Geometry: final body of the model. Coordinates: model frame, mm. A direction names the side the tool comes from. Give positions to 0.01 mm unless a question says otherwise; leave off trailing zeros. Loops run counter-clockwise (first coordinate to the right, second up) from the corner with the lowest first, then second, coordinate; pieces in that order, holes last.
Autodesk Inventor part; units mm, degrees
ref_plane "YZ Plane" through (0, 0, 0) normal (1, 0, 0) x (0, 1, 0)
ref_plane "XZ Plane" through (0, 0, 0) normal (0, 1, 0) x (-1, 0, 0)
ref_plane "XY Plane" through (0, 0, 0) normal (0, 0, 1) x (1, 0, 0)
sketch "Sketch1" plane through (0, 0, 0) normal (1, 0, 0) x (0, 1, 0)
  circle A0 centre (0, 0) radius 50.8
  circle A1 centre (0, 0) radius 3.175
  circle A2 centre (0, -31.75) radius 9.525
  line L0 (0, 0) -> (0, -74.7092) construction
  circle A3 centre (27.4963, -15.875) radius 9.525
  circle A4 centre (27.4963, 15.875) radius 9.525
  circle A5 centre (0, 31.75) radius 9.525
  circle A6 centre (-27.4963, 15.875) radius 9.525
  circle A7 centre (-27.4963, -15.875) radius 9.525
  circle A8 centre (0, -12.7) radius 3.175
  circle A9 centre (12.7, 0) radius 3.175
  circle A10 centre (0, 12.7) radius 3.175
  circle A11 centre (-12.7, 0) radius 3.175
  dimension "d0" = 101.6
  dimension "d1" = 6.35
  dimension "d2" = 19.05
  dimension "d3" = 31.75
  dimension "d6" = 360
  dimension "d16" = 6.35
  dimension "d17" = 12.7
  dimension "d24" = 360
extrude "Extrusion3" add sketch "Sketch1" along normal blind 12.7
sketch "Sketch4" plane through (0, 0, 0) normal (-1, 0, 0) x (0, 0, 1)
  circle A0 centre (0, 0) radius 6.35
  circle A1 centre (0, 0) radius 3.175
  dimension "d28" = 12.7
  dimension "d31" = 6.35
extrude "Extrusion5" add sketch "Sketch4" along normal blind 6.35
sketch "Sketch5" plane through (0, 0, 0) normal (0, 1, 0) x (-1, 0, 0)
  circle A0 centre (3.175, 0) radius 1.5875
  line L0 (0, 0) -> (21.9133, 0) construction
  line L1 (6.35, -6.35) -> (6.35, 6.35) construction
  dimension "d34" = 3.175
  dimension "d35" = 3.175
extrude "Extrusion6" cut sketch "Sketch5" along normal through all
properties part number "ShoulderGearYZ"
Item 1: Draft query along Z for faces 1 (the face through (-6.35, 3, -2)), 2 (the face through (6.261, -37.012, 15.456)), 3 (the face through (6.261, -11.012, 49.592)). Return one class per face: +Z half, -Z half, draft (parallel to the pull), parting line (faces both ways), or undercut.
Values follow:
face 1: draft
face 2: undercut
face 3: parting line
Item 2: Ray query, probe 1 along Z at (x, y) = (5, 0) (3 decimals); probe 2 along Z at (x, y) = (1.25, -34); probe 3 along Y at (x, z) = (3.25, -7.5). Return the intervals inside material, ascending.
Values follow:
probe 1: z = -50.8 to -41.275, -22.225 to -15.875, -9.525 to -3.175, 3.175 to 9.525, 15.875 to 22.225, 41.275 to 50.8
probe 2: z = -37.74 to -22.83, -8.92 to 8.92, 22.83 to 37.74
probe 3: y = -50.24 to -32.03, -22.96 to 22.96, 32.03 to 50.24
Item 3: Section query A-A on x = 3.75. Give the number of separate pieces and of enclosed holes in the cut face, plus the area to 3 significant figures.
Values follow:
separate pieces: 1
enclosed holes: 11
area: 6,240 mm2
Item 4: Section query C-C on z = 31.75. Return loops of the section in (x, y) (3 decimals), plus the area to 3 significant figures.
Values follow:
outline: (0, -39.656) - (12.7, -39.656) - (12.7, -9.525) - (0, -9.525) - close; (0, 9.525) - (12.7, 9.525) - (12.7, 39.656) - (0, 39.656) - close
area: 765 mm2
Item 5: Section query B-B on y = -22.5. Return loops of the section in (x, z).
Values follow:
outline: (0, -45.55) - (12.7, -45.55) - (12.7, -23.98) - (0, -23.98) - close; (0, -7.77) - (12.7, -7.77) - (12.7, 7.77) - (0, 7.77) - close; (0, 23.98) - (12.7, 23.98) - (12.7, 45.55) - (0, 45.55) - close
Item 6: Set-up query: faces 4 (the face through (-3.1, -6.3, -0.8)), 5 (the face through (6.26, 9.53, -0.14)), 6 (the face through (-4.64, 4.52, 0.61)). Return all of +Z, -Z, +X, -X, +Y, -Y with unobstructed straight access to the full face (end or side cutting, diameter ignored); none if empty.
Values follow:
face 4: -X
face 5: +X, -X
face 6: +Y
Item 7: Section query D-D on y = 12.7. Return loops of the section in (x, z) (3 decimals), plus the area to 3 significant figures.
Values follow:
outline: (0, -49.187) - (12.7, -49.187) - (12.7, -3.175) - (0, -3.175) - close; (0, 3.175) - (12.7, 3.175) - (12.7, 49.187) - (0, 49.187) - close
area: 1,170 mm2
Item 8: Pin query (flat end, axial travel): pin 1 (5 mm diameter, centred on x = -2, z = -40.5, fed in from +Y); pin 2 (10 mm diameter, centred on x = 3.5, y = -33.5, fed in from +Z); pin 3 (10 mm diameter, centred on x = 4, y = 11.5, fed in from -Z). Return the tip coordinate at first contact, or that it passes through.
Values follow:
pin 1: stops at y = 32.55
pin 2: stops at z = 42.05
pin 3: stops at z = -50.38
